from build123d import *

# Parameters (mm, degrees)
SKETCH_2_W               = 79
SKETCH_2_H               = 50
EXTRUDE_1_DEPTH          = 4
SKETCH_3_R               = 5
SKETCH_3_R_2             = 1.65
EXTRUDE_2_DEPTH          = 4
SKETCH_4_W               = 19.2
SKETCH_4_H               = 25.2
SKETCH_4_W_2             = 16
SKETCH_4_H_2             = 22
EXTRUDE_3_DEPTH          = 6
SKETCH_5_R               = 1.1
EXTRUDE_4_DEPTH          = 2
SKETCH_6_R               = 1.15
CUT_EXTRUDE_1_DEPTH      = 2
SKETCH_7_R               = 1.5
CUT_EXTRUDE_2_DEPTH      = 69
SKETCH_8_R               = 1.65
CUT_EXTRUDE_3_DEPTH      = 5
CUT_EXTRUDE_4_DEPTH      = 10
CUT_EXTRUDE_4_DEPTH_BACK = 0.7


with BuildPart() as part:
    # 草图2 → 凸台-拉伸1 (new body)
    with BuildSketch(Plane(origin=(0, 0, 0), x_dir=(0, 0, -1), z_dir=(1, 0, 0))):
        Rectangle(SKETCH_2_W, SKETCH_2_H)
    extrude(amount=EXTRUDE_1_DEPTH)

    # 草图3 → 凸台-拉伸2 (add)
    with BuildSketch(Plane.XY.offset(39.5)):
        with BuildLine():
            Line((-52.862197769, 14.724395537), (0, 25))
            Line((0, 25), (0, -25))
            Line((0, -25), (-52.862197769, -14.724395537))
            ThreePointArc((-52.862197769, -14.724395537), (-65, 0), (-52.862197769, 14.724395537))
        make_face()
        with Locations((-50, 0)):
            Circle(SKETCH_3_R, mode=Mode.SUBTRACT)
        with Locations((-55.625, 5.625)):
            Circle(SKETCH_3_R_2, mode=Mode.SUBTRACT)
        with Locations((-44.375, 5.625)):
            Circle(SKETCH_3_R_2, mode=Mode.SUBTRACT)
        with Locations((-44.375, -5.625)):
            Circle(SKETCH_3_R_2, mode=Mode.SUBTRACT)
        with Locations((-55.625, -5.625)):
            Circle(SKETCH_3_R_2, mode=Mode.SUBTRACT)
    extrude_2 = extrude(amount=-EXTRUDE_2_DEPTH)

    # 镜向1: 凸台-拉伸2 across plane
    add(extrude_2.mirror(Plane.XY))

    # 草图4 → 凸台-拉伸3 (add)
    with BuildSketch(Plane.ZY):
        Rectangle(SKETCH_4_W, SKETCH_4_H)
        Rectangle(SKETCH_4_W_2, SKETCH_4_H_2, mode=Mode.SUBTRACT)
    extrude(amount=EXTRUDE_3_DEPTH)

    # 草图5 → 凸台-拉伸4 (add)
    with BuildSketch(Plane.ZY.offset(6)):
        with BuildLine():
            Line((12, 9.25), (9.6, 9.25))
            Line((9.6, 9.25), (9.6, 4.75))
            Line((9.6, 4.75), (12, 4.75))
            ThreePointArc((12, 4.75), (14.25, 7), (12, 9.25))
        make_face()
        with Locations((12, 7)):
            Circle(SKETCH_5_R, mode=Mode.SUBTRACT)
        with BuildLine():
            Line((9.6, -9.25), (9.6, -4.75))
            Line((9.6, -4.75), (12, -4.75))
            ThreePointArc((12, -4.75), (14.25, -7), (12, -9.25))
            Line((12, -9.25), (9.6, -9.25))
        make_face()
        with Locations((12, -7)):
            Circle(SKETCH_5_R, mode=Mode.SUBTRACT)
        with BuildLine():
            Line((-12, -9.25), (-9.6, -9.25))
            Line((-9.6, -9.25), (-9.6, -4.75))
            Line((-9.6, -4.75), (-12, -4.75))
            ThreePointArc((-12, -4.75), (-14.25, -7), (-12, -9.25))
        make_face()
        with Locations((-12, -7)):
            Circle(SKETCH_5_R, mode=Mode.SUBTRACT)
        with BuildLine():
            Line((-9.6, 9.25), (-9.6, 4.75))
            Line((-9.6, 4.75), (-12, 4.75))
            ThreePointArc((-12, 4.75), (-14.25, 7), (-12, 9.25))
            Line((-12, 9.25), (-9.6, 9.25))
        make_face()
        with Locations((-12, 7)):
            Circle(SKETCH_5_R, mode=Mode.SUBTRACT)
    extrude(amount=-EXTRUDE_4_DEPTH)

    # 草图6 → 切除-拉伸1 (cut)
    with BuildSketch(Plane.XY.offset(-8)):
        with Locations((-6, 0)):
            Circle(SKETCH_6_R)
    extrude(amount=-CUT_EXTRUDE_1_DEPTH, mode=Mode.SUBTRACT)

    # 草图7 → 切除-拉伸2 (cut)
    with BuildSketch(Plane(origin=(-12.802515134, 0, -6.523207278), x_dir=(0, 1, 0), z_dir=(0.891006524, 0, 0.4539905))):
        with Locations((0, -19.010719704)):
            Circle(SKETCH_7_R)
    extrude(amount=-CUT_EXTRUDE_2_DEPTH, mode=Mode.SUBTRACT)

    # 草图8 → 切除-拉伸3 (cut, through all)
    with BuildSketch(Plane.ZY):
        with Locations((-33, 17.5)):
            Circle(SKETCH_8_R)
        with Locations((22, 17.5)):
            Circle(SKETCH_8_R)
        with Locations((22, -17.5)):
            Circle(SKETCH_8_R)
        with Locations((-33, -17.5)):
            Circle(SKETCH_8_R)
    extrude(amount=-CUT_EXTRUDE_3_DEPTH, mode=Mode.SUBTRACT)

    # 草图9 → 切除-拉伸4 (cut, two sides)
    with BuildSketch(Plane.ZY) as cut_extrude_4_sk:
        Polygon((-31.383419246, 14.7), (-29.766838493, 17.5), (-31.383419246, 20.3), (-34.616580754, 20.3), (-36.233161507, 17.5), (-34.616580754, 14.7), align=None)
        Polygon((-29.766838493, -17.5), (-31.383419246, -14.7), (-34.616580754, -14.7), (-36.233161507, -17.5), (-34.616580754, -20.3), (-31.383419246, -20.3), align=None)
        Polygon((23.616580754, -14.7), (20.383419246, -14.7), (18.766838493, -17.5), (20.383419246, -20.3), (23.616580754, -20.3), (25.233161507, -17.5), align=None)
        Polygon((25.233161507, 17.5), (23.616580754, 20.3), (20.383419246, 20.3), (18.766838493, 17.5), (20.383419246, 14.7), (23.616580754, 14.7), align=None)
    extrude(amount=CUT_EXTRUDE_4_DEPTH, mode=Mode.SUBTRACT)
    extrude(cut_extrude_4_sk.sketch, amount=-CUT_EXTRUDE_4_DEPTH_BACK, mode=Mode.SUBTRACT)


solid = part.part
Read the model definition and answer for the solid it produces. Units are mm, in the model's axes. A direction names the side the tool comes from. Give positions to 0.01 mm unless a question says otherwise; leave off trailing zeros. Write each loop counter-clockwise with the first axis right and the second up, starting at its lowest first coordinate (ties: lowest second). Pieces come first, ordered by that corner, then holes. Notation, with made-up numbers: M 13.5,47.5 L 36.5,47.5 A20 cw 36.5,58.5 Z; hole C 0,85 d1. An arc over 180 degrees is marked long. One line per item, written item: value. Start each with the question number.
(1) Find section B-B (x = -48). Determine the outline of the cut face in (y, z).
(2) Find section D-D (z = 6.5). Determine the outline of the cut face in (x, y).
(3) Find section A-A (z = 22). Determine the outline of the cut face in (x, y), plus the area to 3 significant figures.
(4) Find section C-C (y = 0). Determine the outline of the cut face in (x, z).
(5) Determine the mould class of faces 6 (the flat face through (-3, 12.6, 0)), 7 (the flat face through (0.7, 19, 23)), 8 (the flat face through (-25, 0, 35.5)), 9 (the flat face through (-3, -12.6, 0)) for opening direction Y: pulls with the +Y half, pulls with the -Y half, needs draft (parallel to the pull), parting line crosses it, or undercut.
(6) Flat-ended cylindrical pins translate along their axes: pin 1 Ø1.3 at (y, z) = (7, 12) entering from -X; pin 2 Ø2.5 at (y, z) = (-7, -12) entering from -X; pin 3 Ø12 at (x, y) = (-48, -17) entering from +Z; pin 4 Ø4.5 at (y, z) = (-17.5, 22.5) entering from -X. Find the tip coordinate at first contact, or state that the pin passes through.
(7) Find the intervals of material crossed by line 1 (Z direction, x = -36, y = 15); line 2 (Y direction, x = -4.7, z = -12); line 3 (Z direction, x = -1.5, y = 1), in increasing order.
(8) A tool of negligible diameter and unlimited length cuts with its end or side. For faces 1 (the flat face through (-5, -9.25, 11)), 2 (the flat face through (-4, 8, 11)), 3 (the flat face through (-5, 4.75, 11)), 4 (the flat face through (-2, 0, -9.6)), 5 (the flat face through (-5, 9.25, -11)), from which of +Z, -Z, +X, -X, +Y, -Y can it reach the whole face along a straight path? Write none if from no direction.
Results below:
1. outline: M -15.67,-39.5 L -4.58,-39.5 L -4.58,-35.5 L -15.67,-35.5 Z; M -15.67,35.5 L -4.58,35.5 L -4.58,39.5 L -15.67,39.5 Z; M 4.58,-39.5 L 15.67,-39.5 L 15.67,-35.5 L 4.58,-35.5 Z; M 4.58,35.5 L 15.67,35.5 L 15.67,39.5 L 4.58,39.5 Z
2. outline: M -6,-12.6 L 0,-12.6 L 0,-25 L 4,-25 L 4,25 L 0,25 L 0,12.6 L -6,12.6 L -6,11 L 0,11 L 0,-11 L -6,-11 Z
3. outline: M 0,-25 L 4,-25 L 4,-19.15 L 0.7,-19.15 L 0.7,-20.3 L 0,-20.3 Z; M 0,-14.7 L 0.7,-14.7 L 0.7,-15.85 L 4,-15.85 L 4,15.85 L 0.7,15.85 L 0.7,14.7 L 0,14.7 Z; M 0,20.3 L 0.7,20.3 L 0.7,19.15 L 4,19.15 L 4,25 L 0,25 Z
3. area: 170 mm^2
4. outline: M -65,-39.5 L -55,-39.5 L -55,-35.5 L -65,-35.5 Z; M -65,35.5 L -55,35.5 L -55,39.5 L -65,39.5 Z; M -45,-39.5 L -38.95,-39.5 L -31.1,-35.5 L -45,-35.5 Z; M -45,35.5 L 0,35.5 L 0,9.6 L -6,9.6 L -6,8 L 0,8 L 0,-8 L -4.85,-8 L -4.85,-9.6 L 0,-9.6 L 0,-35.5 L -24.49,-35.5 L -32.34,-39.5 L 4,-39.5 L 4,39.5 L -45,39.5 Z
5. face 6: pulls with the +Y half
5. face 7: undercut
5. face 8: needs draft
5. face 9: pulls with the -Y half
6. pin 1: stops at x = 0
6. pin 2: stops at x = -6
6. pin 3: stops at z = 39.5
6. pin 4: stops at x = 0.7
7. line 1: z = -39.5 to -35.5, 35.5 to 39.5
7. line 2: y = -9.25 to -8.1, -5.9 to -4.75, 4.75 to 5.9, 8.1 to 9.25
7. line 3: z = -39.5 to -35.5, -9.6 to -8, 8 to 9.6, 35.5 to 39.5
8. face 1: -X, -Y
8. face 2: +Y, -Y
8. face 3: -X
8. face 4: none
8. face 5: -X, +Y
